Source: CAD feature listing. Evaluate the final solid. Frame: model axes, mm. A direction names the side the tool comes from. Coordinates: 2 decimals unless noted, no trailing zeros. Order: outer loops, then holes, each group sorted by start corner. A loop starts at its lowest first (then second) coordinate and runs counter-clockwise, first axis right, second up.
```python
from build123d import *

# Parameters (mm, degrees)
EKSTR_ZYON_NCE1_DEPTH = 60
RADYUS1_R             = 10
KES_EKSTR_ZYON3_REACH = 133.651
IZIM3_R               = 2.5
KES_EKSTR_ZYON4_REACH = 135.342
IZIM4_R               = 2
IZIM4_W               = 40
IZIM4_H               = 20
KES_EKSTR_ZYON5_REACH = 135.342
IZIM5_R               = 4


with BuildPart() as part:
    # Çizim1 → Ekstrüzyon-İnce1 (new body)
    with BuildSketch(Plane.XY):
        Polygon((0, 0), (100, 0), (100, 50), (0, 50), (0, 54), (104, 54), (104, -4), (0, -4), align=None)
    extrude(amount=EKSTR_ZYON_NCE1_DEPTH)

    # Radyus1
    radyus1_edges = [part.edges().sort_by_distance(p)[0] for p in [
        (0, -2, 60),
        (0, 52, 60),
        (0, -2, 0),
        (0, 52, 0),
    ]]
    fillet(radyus1_edges, radius=RADYUS1_R)

    # Çizim3 → Kes-Ekstrüzyon3 (cut, up to next)
    with BuildSketch(Plane(origin=(104, 0, 0), x_dir=(0, 0, -1), z_dir=(1, 0, 0)), mode=Mode.PRIVATE) as kes_ekstr_zyon3_sk1:
        with Locations((-30, 40)):
            Circle(IZIM3_R)
    kes_ekstr_zyon3_tool1 = extrude(kes_ekstr_zyon3_sk1.sketch, amount=-KES_EKSTR_ZYON3_REACH, mode=Mode.PRIVATE) & part.part
    # Çizim3 → Kes-Ekstrüzyon3 (cut, up to next)
    with BuildSketch(Plane(origin=(104, 0, 0), x_dir=(0, 0, -1), z_dir=(1, 0, 0)), mode=Mode.PRIVATE) as kes_ekstr_zyon3_sk2:
        with Locations(Location((-30, 10, 0), (0, 0, 180))):
            Circle(IZIM3_R)
    kes_ekstr_zyon3_tool2 = extrude(kes_ekstr_zyon3_sk2.sketch, amount=-KES_EKSTR_ZYON3_REACH, mode=Mode.PRIVATE) & part.part
    # Çizim3 → Kes-Ekstrüzyon3 (cut, up to next)
    with BuildSketch(Plane(origin=(104, 0, 0), x_dir=(0, 0, -1), z_dir=(1, 0, 0)), mode=Mode.PRIVATE) as kes_ekstr_zyon3_sk3:
        with Locations((-15, 25)):
            Circle(IZIM3_R)
    kes_ekstr_zyon3_tool3 = extrude(kes_ekstr_zyon3_sk3.sketch, amount=-KES_EKSTR_ZYON3_REACH, mode=Mode.PRIVATE) & part.part
    # Çizim3 → Kes-Ekstrüzyon3 (cut, up to next)
    with BuildSketch(Plane(origin=(104, 0, 0), x_dir=(0, 0, -1), z_dir=(1, 0, 0)), mode=Mode.PRIVATE) as kes_ekstr_zyon3_sk4:
        with Locations(Location((-45, 25, 0), (0, 0, 180))):
            Circle(IZIM3_R)
    kes_ekstr_zyon3_tool4 = extrude(kes_ekstr_zyon3_sk4.sketch, amount=-KES_EKSTR_ZYON3_REACH, mode=Mode.PRIVATE) & part.part
    add(kes_ekstr_zyon3_tool1.solids().sort_by_distance((104, 40, 30))[0], mode=Mode.SUBTRACT)
    add(kes_ekstr_zyon3_tool2.solids().sort_by_distance((104, 10, 30))[0], mode=Mode.SUBTRACT)
    add(kes_ekstr_zyon3_tool3.solids().sort_by_distance((104, 25, 15))[0], mode=Mode.SUBTRACT)
    add(kes_ekstr_zyon3_tool4.solids().sort_by_distance((104, 25, 45))[0], mode=Mode.SUBTRACT)

    # Çizim4 → Kes-Ekstrüzyon4 (cut, up to next)
    with BuildSketch(Plane(origin=(0, 54, 0), x_dir=(1, 0, 0), z_dir=(0, 1, 0)), mode=Mode.PRIVATE) as kes_ekstr_zyon4_sk1:
        with Locations(Location((26.5, -25, 0), (0, 0, 180))):
            Circle(IZIM4_R)
    kes_ekstr_zyon4_tool1 = extrude(kes_ekstr_zyon4_sk1.sketch, amount=-KES_EKSTR_ZYON4_REACH, mode=Mode.PRIVATE) & part.part
    # Çizim4 → Kes-Ekstrüzyon4 (cut, up to next)
    with BuildSketch(Plane(origin=(0, 54, 0), x_dir=(1, 0, 0), z_dir=(0, 1, 0)), mode=Mode.PRIVATE) as kes_ekstr_zyon4_sk2:
        with Locations((26.5, -35)):
            Circle(IZIM4_R)
    kes_ekstr_zyon4_tool2 = extrude(kes_ekstr_zyon4_sk2.sketch, amount=-KES_EKSTR_ZYON4_REACH, mode=Mode.PRIVATE) & part.part
    # Çizim4 → Kes-Ekstrüzyon4 (cut, up to next)
    with BuildSketch(Plane(origin=(0, 54, 0), x_dir=(1, 0, 0), z_dir=(0, 1, 0)), mode=Mode.PRIVATE) as kes_ekstr_zyon4_sk3:
        with Locations(Location((73.5, -35, 0), (0, 0, 180))):
            Circle(IZIM4_R)
    kes_ekstr_zyon4_tool3 = extrude(kes_ekstr_zyon4_sk3.sketch, amount=-KES_EKSTR_ZYON4_REACH, mode=Mode.PRIVATE) & part.part
    # Çizim4 → Kes-Ekstrüzyon4 (cut, up to next)
    with BuildSketch(Plane(origin=(0, 54, 0), x_dir=(1, 0, 0), z_dir=(0, 1, 0)), mode=Mode.PRIVATE) as kes_ekstr_zyon4_sk4:
        with Locations((73.5, -25)):
            Circle(IZIM4_R)
    kes_ekstr_zyon4_tool4 = extrude(kes_ekstr_zyon4_sk4.sketch, amount=-KES_EKSTR_ZYON4_REACH, mode=Mode.PRIVATE) & part.part
    # Çizim4 → Kes-Ekstrüzyon4 (cut, up to next)
    with BuildSketch(Plane(origin=(0, 54, 0), x_dir=(1, 0, 0), z_dir=(0, 1, 0)), mode=Mode.PRIVATE) as kes_ekstr_zyon4_sk5:
        with Locations((50, -30)):
            Rectangle(IZIM4_W, IZIM4_H)
    kes_ekstr_zyon4_tool5 = extrude(kes_ekstr_zyon4_sk5.sketch, amount=-KES_EKSTR_ZYON4_REACH, mode=Mode.PRIVATE) & part.part
    add(kes_ekstr_zyon4_tool1.solids().sort_by_distance((26.5, 54, 25))[0], mode=Mode.SUBTRACT)
    add(kes_ekstr_zyon4_tool2.solids().sort_by_distance((26.5, 54, 35))[0], mode=Mode.SUBTRACT)
    add(kes_ekstr_zyon4_tool3.solids().sort_by_distance((73.5, 54, 35))[0], mode=Mode.SUBTRACT)
    add(kes_ekstr_zyon4_tool4.solids().sort_by_distance((73.5, 54, 25))[0], mode=Mode.SUBTRACT)
    add(kes_ekstr_zyon4_tool5.solids().sort_by_distance((50, 54, 30))[0], mode=Mode.SUBTRACT)

    # Çizim5 → Kes-Ekstrüzyon5 (cut, up to next)
    with BuildSketch(Plane.XZ.offset(4), mode=Mode.PRIVATE) as kes_ekstr_zyon5_sk1:
        with Locations(Location((40, 30, 0), (0, 0, 270))):
            Circle(IZIM5_R)
    kes_ekstr_zyon5_tool1 = extrude(kes_ekstr_zyon5_sk1.sketch, amount=-KES_EKSTR_ZYON5_REACH, mode=Mode.PRIVATE) & part.part
    # Çizim5 → Kes-Ekstrüzyon5 (cut, up to next)
    with BuildSketch(Plane.XZ.offset(4), mode=Mode.PRIVATE) as kes_ekstr_zyon5_sk2:
        with Locations(Location((60, 30, 0), (0, 0, 270))):
            Circle(IZIM5_R)
    kes_ekstr_zyon5_tool2 = extrude(kes_ekstr_zyon5_sk2.sketch, amount=-KES_EKSTR_ZYON5_REACH, mode=Mode.PRIVATE) & part.part
    add(kes_ekstr_zyon5_tool1.solids().sort_by_distance((40, -4, 30))[0], mode=Mode.SUBTRACT)
    add(kes_ekstr_zyon5_tool2.solids().sort_by_distance((60, -4, 30))[0], mode=Mode.SUBTRACT)


solid = part.part
```
Q1. Pull-direction query (X, two-part tool) for faces 4 (the flat face through (30, 52, 30)), 5 (the flat face through (0, -2, 30)), 6 (the cylindrical face through (102.03, 22.89, 46.34)); classes: pulls with the +X half, pulls with the -X half, needs draft (parallel to the pull), parting line crosses it, or undercut.
Solutions:
face 4: undercut
face 5: pulls with the -X half
face 6: needs draft
Q2. Section query D-D on z = 30. Output: boundary loops of the cut face in (x, y).
Solutions:
outline: (0, -4) - (36, -4) - (36, 0) - (0, 0) - close; (0, 50) - (30, 50) - (30, 54) - (0, 54) - close; (44, -4) - (56, -4) - (56, 0) - (44, 0) - close; (64, -4) - (104, -4) - (104, 7.5) - (100, 7.5) - (100, 0) - (64, 0) - close; (70, 50) - (100, 50) - (100, 42.5) - (104, 42.5) - (104, 54) - (70, 54) - close; (100, 12.5) - (104, 12.5) - (104, 37.5) - (100, 37.5) - close
Q3. Pin query (flat end, axial travel): P1, Ø4, axis at y = 10, z = 30, coming from the +X side (1 decimal); P2, Ø3, axis at x = 42, z = 37, coming from the +Y side. Return the tip coordinate at first contact, or that it passes through.
Solutions:
P1: passes through
P2: stops at y = 0
Q4. Material intervals for line 1 along Z through (x, y) = (73.5, 52.5); line 2 along Y through (x, z) = (102.15, 30); line 3 along Y through (x, z) = (27.5, 12), sorted ascending.
Solutions:
line 1: z = 0 to 23, 27 to 33, 37 to 60
line 2: y = -4 to 7.5, 12.5 to 37.5, 42.5 to 54
line 3: y = -4 to 0, 50 to 54
Q5. Section query A-A on x = 68. Output: boundary loops of the cut face in (y, z).
Solutions:
outline: (-4, 0) - (0, 0) - (0, 60) - (-4, 60) - close; (50, 0) - (54, 0) - (54, 20) - (50, 20) - close; (50, 40) - (54, 40) - (54, 60) - (50, 60) - close
Q6. Section query B-B on y = 10. Output: boundary loops of the cut face in (x, z).
Solutions:
outline: (100, 0) - (104, 0) - (104, 27.5) - (100, 27.5) - close; (100, 32.5) - (104, 32.5) - (104, 60) - (100, 60) - close
Q7. Set-up query: faces 1 (the cylindrical face through (25.577, 52.028, 23.226)), 2 (the flat face through (64, -1, 0)), 3 (the flat face through (100, 25, 30)). Return all of +Z, -Z, +X, -X, +Y, -Y with unobstructed straight access to the full face (end or side cutting, diameter ignored); none if empty.
Solutions:
face 1: +Y
face 2: -Z, +X, -X, +Y, -Y
face 3: +Z, -Z, -X
Q8. Section query C-C on x = 40. Output: boundary loops of the cut face in (y, z), plus the area to 3 significant figures.
Solutions:
outline: (-4, 0) - (0, 0) - (0, 26) - (-4, 26) - close; (-4, 34) - (0, 34) - (0, 60) - (-4, 60) - close; (50, 0) - (54, 0) - (54, 20) - (50, 20) - close; (50, 40) - (54, 40) - (54, 60) - (50, 60) - close
area: 368 mm2
